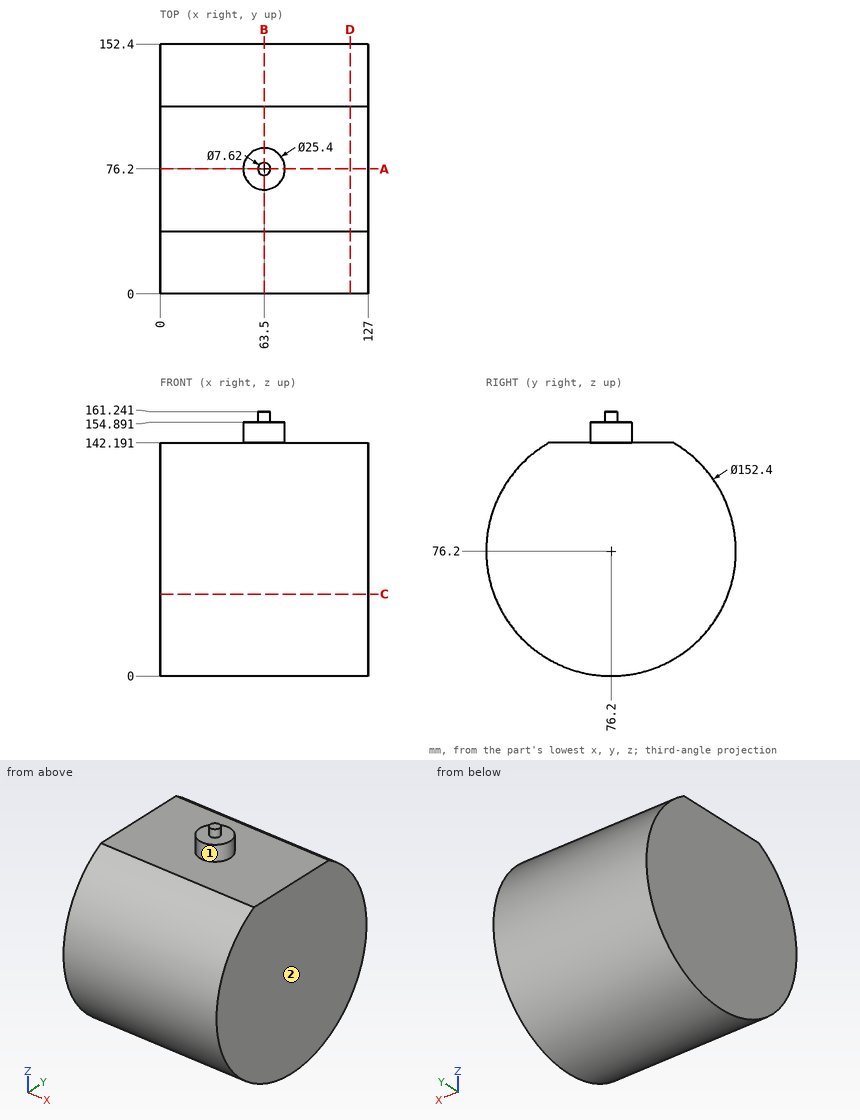
For this review, use the dimensioned drawing (mm, ordinates from the lowest corner) and the shaded views. A direction names the side the tool comes from. Round coordinates to 2 decimals unless told otherwise and drop trailing zeros. Order: outer loops, then holes, each group sorted by start corner. A loop starts at its lowest first (then second) coordinate and runs counter-clockwise, first axis right, second up. Notation, with made-up numbers: M 28.25,-8.5 L 62.25,-8.5 A17 ccw 62.25,-2.5 Z; hole C 20,84 d1. An arc over 180 degrees is marked long. Write each question's results on one line, items separated by ' | '. Start each with the question number.
1. Add section C-C (z = 50). State the section outline as (x, y) points.
2. Tool access review of the marked faces 1 and 2: name each direction out of +Z, -Z, +X, -X, +Y, -Y from which nothing blocks a thin tool from reaching the whole face with its end or side.
3. Add section D-D (x = 116). State the section outline as (y, z) points, then the cut area to 3 significant figures.
4. Add section B-B (x = 63.5). State the section outline as (y, z) points, then the cut area to 3 significant figures.
5. Add section A-A (y = 76.2). State the section outline as (x, z) points, then the cut area to 3 significant figures.
6. Clearance check with flat-ended pins moving along their axes: pin 1 Ø2 at (x, z) = (112, 95) entering from +Y; pin 2 Ø5 at (x, y) = (40, 51) entering from +Z; pin 3 Ø3 at (x, y) = (17, 132.5) entering from +Z. State where each tip first meets the part, or that it passes through.
7. To check wall thickness, follow L1, parallel to Y at x = 117, z = 76.5; L2, parallel to Z at x = 15, y = 77; L3, parallel to Z at x = 113, y = 26. State the ranges of each line that lie inside material, in increasing order. Write a range as [from, to].
Output values:
1) outline: M 0,4.65 L 127,4.65 L 127,147.75 L 0,147.75 Z
2) face 1: +Z | face 2: +Z, -Z, +X, +Y, -Y
3) outline: M 38.1,142.19 A76.2 ccw long 114.3,142.19 Z | area: 17,700 mm^2
4) outline: M 38.1,142.19 A76.2 ccw long 114.3,142.19 L 88.9,142.19 L 88.9,154.89 L 80.01,154.89 L 80.01,161.24 L 72.39,161.24 L 72.39,154.89 L 63.5,154.89 L 63.5,142.19 Z | area: 18,100 mm^2
5) outline: M 0,0 L 127,0 L 127,142.19 L 76.2,142.19 L 76.2,154.89 L 67.31,154.89 L 67.31,161.24 L 59.69,161.24 L 59.69,154.89 L 50.8,154.89 L 50.8,142.19 L 0,142.19 Z | area: 18,400 mm^2
6) pin 1: y = 150.29 | pin 2: z = 142.19 | pin 3: z = 129.15
7) L1: [0, 152.4] | L2: [0, 142.19] | L3: [18.87, 133.53]
